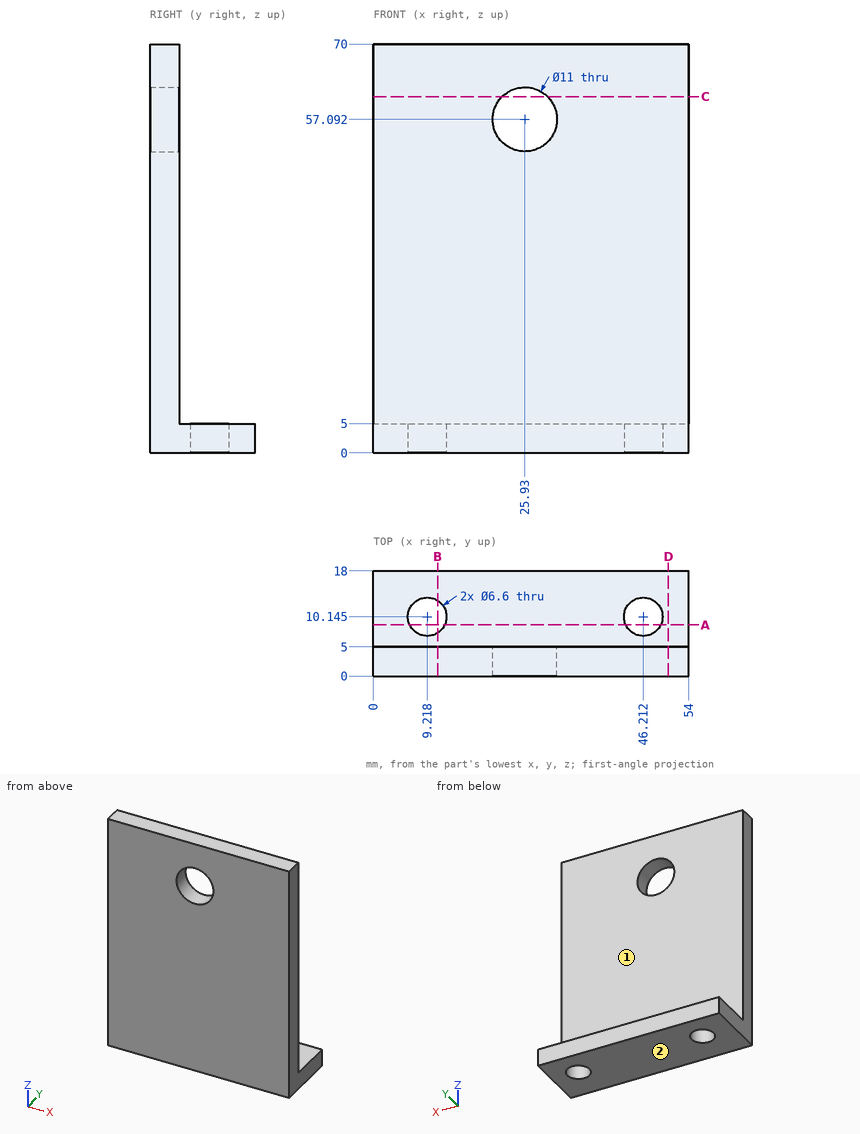
Answer from the drawing. Dimensions are ordinates in mm from the lowest x, y and z of the part. A direction names the side the tool comes from. Round coordinates to 2 decimals unless told otherwise and drop trailing zeros. Order: outer loops, then holes, each group sorted by start corner. A loop starts at its lowest first (then second) coordinate and runs counter-clockwise, first axis right, second up.
1) The part is cut by section D-D on x = 50.5. Write down the section's boundary in (y, z), plus the area to 3 significant figures.
2) The part is cut by section C-C on z = 61. Write down the section's boundary in (x, y), plus the area to 3 significant figures.
3) The part is cut by section A-A on y = 8.75. Write down the section's boundary in (x, z).
4) Straight lines are drawn through the part: L1, parallel to X at y = 2.5, z = 57; L2, parallel to Z at x = 37, y = 7. For each, find the intervals that lie inside material, in ascending order.
5) The part is cut by section B-B on x = 11. Write down the section's boundary in (y, z).
6) For the marked faces 1 and 2, determine the directions among +Z, -Z, +X, -X, +Y, -Y from which every point of the face is accessible in a straight line to the end or side of a thin tool.
7) Flat-ended cylindrical pins translate along their axes: pin 1 (1 mm diameter, centred on x = 44, z = 35.5, fed in from +Y); pin 2 (1 mm diameter, centred on x = 38, z = 45, fed in from -Y); pin 3 (7.5 mm diameter, centred on x = 46.21, y = 10.14, fed in from +Z). Find the tip coordinate at first contact, or state that the pin passes through.
Resolved:
1. outline: (0, 0) - (18, 0) - (18, 5) - (5, 5) - (5, 70) - (0, 70) - close
1. area: 415 mm2
2. outline: (0, 0) - (22.06, 0) - (22.06, 5) - (0, 5) - close; (29.8, 0) - (54, 0) - (54, 5) - (29.8, 5) - close
2. area: 231 mm2
3. outline: (0, 0) - (6.23, 0) - (6.23, 5) - (0, 5) - close; (12.21, 0) - (43.22, 0) - (43.22, 5) - (12.21, 5) - close; (49.2, 0) - (54, 0) - (54, 5) - (49.2, 5) - close
4. L1: x = 0 to 20.43, 31.43 to 54
4. L2: z = 0 to 5
5. outline: (0, 0) - (7.37, 0) - (7.37, 5) - (5, 5) - (5, 70) - (0, 70) - close; (12.92, 0) - (18, 0) - (18, 5) - (12.92, 5) - close
6. face 1: +Z, +X, -X, +Y
6. face 2: -Z, +X, -X, +Y, -Y
7. pin 1: stops at y = 5
7. pin 2: stops at y = 0
7. pin 3: stops at z = 5
